Geometry check sheet. Reference: the model listing, model coordinates, mm. Give positions to 0.01 mm unless a question says otherwise; leave off trailing zeros. Loops run counter-clockwise (first coordinate to the right, second up) from the corner with the lowest first, then second, coordinate; pieces in that order, holes last. Notation, with made-up numbers: (51.5, 77) - (57.5, 77) arc R28 cw to (57.5, 113) - close; hole circle Ø8 at (-40, -34). An arc over 180 degrees is marked (long way). Use a Markdown table: item, result. Add a question column.
1. Material ranges on L1, parallel to Z at x = 1, y = -3.5; L2, parallel to Z at x = 3.5, y = 2.25; L3, parallel to X at y = 1.25, z = -1.75, recorded low to high.
2. Cross-section at C-C on z = -1.5. Enter the section's corners in (x, y), and give its area (3 significant figures).
3. Depth check by flat-ended pin: P1, Ø3, axis at x = 44.5, z = 0, coming from the +Y side. Enter the tip coordinate at first touch or a pass-through.
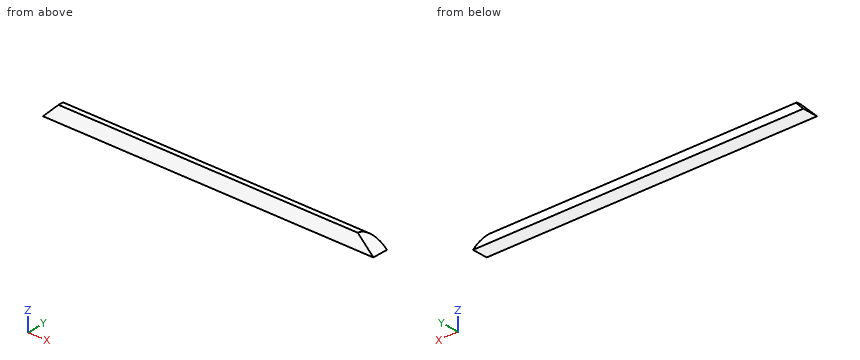
from build123d import *

# Parameters (mm, degrees)
SKETCH002_W     = 170
SKETCH002_H     = 8
PAD002_DEPTH    = 4
CHAMFER001_SIZE = 7.99
FILLET001_R     = 7.99


with BuildPart() as part:
    # Sketch002 → Pad002 (new body, symmetric)
    with BuildSketch(Plane.XZ):
        Rectangle(SKETCH002_W, SKETCH002_H)
    extrude(amount=PAD002_DEPTH, both=True)

    # Chamfer001
    chamfer001_edges = [part.edges().sort_by_distance(p)[0] for p in [
        (85, 0, 4),
        (-85, 0, 4),
    ]]
    chamfer(chamfer001_edges, length=CHAMFER001_SIZE)

    # Fillet001
    fillet001_edges = [part.edges().sort_by_distance(p)[0] for p in [
        (0, 4, 4),
    ]]
    fillet(fillet001_edges, radius=FILLET001_R)


solid = part.part
Values found:
| question | item | result |
|---|---|---|
| 1 | L1 | z = -4 to 3.98 |
| 1 | L2 | z = -4 to 1 |
| 1 | L3 | x = -82.76 to 82.76 |
| 2 | outline | (-82.51, -4) - (82.51, -4) - (82.51, 3.6) - (-82.51, 3.6) - close |
| 2 | area | 1,250 mm2 |
| 3 | P1 | stops at y = 3.6 |
